from build123d import *

# Parameters (mm, degrees)
SZKIC1_W                       = 40
SZKIC1_H                       = 14
SZKIC1_R                       = 2
DODANIE_WYCI_GNI_CIE1_DEPTH    = 10.77
SZKIC2_W                       = 56
SZKIC2_H                       = 14
DODANIE_WYCI_GNI_CIE2_DEPTH    = 20.3
SZKIC5_R                       = 2.25
WYTNIJ_WYCI_GNI_CIE2_DEPTH     = 14
SZKIC8_W                       = 56
SZKIC8_H                       = 10.77
DODANIE_WYCI_GNI_CIE3_DEPTH    = 14
WYTNIJ_WYCI_GNI_CIE3_START     = -14
WYTNIJ_WYCI_GNI_CIE3_OUTLINE_W = 42
WYTNIJ_WYCI_GNI_CIE3_OUTLINE_H = 21
WYTNIJ_WYCI_GNI_CIE3_DEPTH     = 14
SZKIC12_R                      = 2.25
DODANIE_WYCI_GNI_CIE4_DEPTH    = 18
WYTNIJ_WYCI_GNI_CIE1_DEPTH     = 5
SZKIC9_R                       = 2.2
WYTNIJ_WYCI_GNI_CIE4_DEPTH     = 21
SZKIC10_W                      = 56
SZKIC10_H                      = 21
WYTNIJ_WYCI_GNI_CIE5_DEPTH     = 17
SZKIC13_W                      = 21
SZKIC13_H                      = 15
DODANIE_WYCI_GNI_CIE5_DEPTH    = 0.7
SZKIC16_W                      = 21
SZKIC16_H                      = 15
DODANIE_WYCI_GNI_CIE7_DEPTH    = 0.7


# Read off the part's stored shape, not the designer's step: Wytnij-wyciągnięcie3
with BuildPart() as part:
    # Szkic1 → Dodanie-wyciągnięcie1 (new body)
    with BuildSketch(Plane.XY):
        Rectangle(SZKIC1_W, SZKIC1_H)
        with Locations((-14, 0)):
            Circle(SZKIC1_R, mode=Mode.SUBTRACT)
        with Locations((14, 0)):
            Circle(SZKIC1_R, mode=Mode.SUBTRACT)
    extrude(amount=DODANIE_WYCI_GNI_CIE1_DEPTH)

    # Szkic2 → Dodanie-wyciągnięcie2 (add)
    with BuildSketch(Plane.XY.offset(10.77)):
        Rectangle(SZKIC2_W, SZKIC2_H)
    extrude(amount=DODANIE_WYCI_GNI_CIE2_DEPTH)

    # Szkic5 → Wytnij-wyciągnięcie2 (cut)
    with BuildSketch(Plane(origin=(0, 7, 0), x_dir=(1, 0, 0), z_dir=(0, 1, 0))):
        with Locations(Location((-24, -15.92, 0), (0, 0, 180))):
            Circle(SZKIC5_R)
        with Locations(Location((24, -15.92, 0), (0, 0, 180))):
            Circle(SZKIC5_R)
        with Locations(Location((24, -25.92, 0), (0, 0, 180))):
            Circle(SZKIC5_R)
        with Locations(Location((-24, -25.92, 0), (0, 0, 180))):
            Circle(SZKIC5_R)
    extrude(amount=-WYTNIJ_WYCI_GNI_CIE2_DEPTH, mode=Mode.SUBTRACT)

    # Szkic8 → Dodanie-wyciągnięcie3 (add)
    with BuildSketch(Plane(origin=(0, 7, 0), x_dir=(1, 0, 0), z_dir=(0, 1, 0))):
        with Locations((0, -5.385)):
            Rectangle(SZKIC8_W, SZKIC8_H)
    extrude(amount=-DODANIE_WYCI_GNI_CIE3_DEPTH)

    # Wytnij-wyciągnięcie3 outline → Wytnij-wyciągnięcie3 (cut)
    with BuildSketch(Plane(origin=(0, 7, 0), x_dir=(1, 0, 0), z_dir=(0, 1, 0)).offset(WYTNIJ_WYCI_GNI_CIE3_START)):
        with Locations((-0.124911353, -20.57)):
            Rectangle(WYTNIJ_WYCI_GNI_CIE3_OUTLINE_W, WYTNIJ_WYCI_GNI_CIE3_OUTLINE_H)
    extrude(amount=WYTNIJ_WYCI_GNI_CIE3_DEPTH, mode=Mode.SUBTRACT)

    # Szkic12 → Dodanie-wyciągnięcie4 (add)
    with BuildSketch(Plane.XZ.offset(7)):
        Polygon((20.875088647, 31.07), (20.875088647, 10.07), (-21.124911353, 10.07), (-21.124911353, 31.07), (-28, 31.07), (-28, 0), (28, 0), (28, 31.07), align=None)
        with Locations(Location((-24, 25.92, 0), (0, 0, 180))):
            Circle(SZKIC12_R, mode=Mode.SUBTRACT)
        with Locations(Location((24, 25.92, 0), (0, 0, 180))):
            Circle(SZKIC12_R, mode=Mode.SUBTRACT)
        with Locations(Location((-24, 15.92, 0), (0, 0, 180))):
            Circle(SZKIC12_R, mode=Mode.SUBTRACT)
        with Locations(Location((24, 15.92, 0), (0, 0, 180))):
            Circle(SZKIC12_R, mode=Mode.SUBTRACT)
    extrude(amount=DODANIE_WYCI_GNI_CIE4_DEPTH)

    # Szkic4 → Wytnij-wyciągnięcie1 (cut)
    with BuildSketch(Plane.XY.offset(10.77)):
        Polygon((-16.078460969, 3.6), (-18.156921938, 0), (-16.078460969, -3.6), (-11.921539031, -3.6), (-9.843078062, 0), (-11.921539031, 3.6), align=None)
        Polygon((11.921539031, 3.6), (9.843078062, 0), (11.921539031, -3.6), (16.078460969, -3.6), (18.156921938, 0), (16.078460969, 3.6), align=None)
    extrude(amount=-WYTNIJ_WYCI_GNI_CIE1_DEPTH, mode=Mode.SUBTRACT)

    # Szkic9 → Wytnij-wyciągnięcie4 (cut)
    with BuildSketch(Plane.XY.offset(10.07)):
        with Locations((-14, 0)):
            Circle(SZKIC9_R)
        with Locations((14, 0)):
            Circle(SZKIC9_R)
    extrude(amount=-WYTNIJ_WYCI_GNI_CIE4_DEPTH, mode=Mode.SUBTRACT)

    # Szkic10 → Wytnij-wyciągnięcie5 (cut)
    with BuildSketch(Plane(origin=(0, 7, 0), x_dir=(1, 0, 0), z_dir=(0, 1, 0))):
        with Locations((0, -20.57)):
            Rectangle(SZKIC10_W, SZKIC10_H)
    extrude(amount=-WYTNIJ_WYCI_GNI_CIE5_DEPTH, mode=Mode.SUBTRACT)

    # Szkic13 → Dodanie-wyciągnięcie5 (add)
    with BuildSketch(Plane(origin=(-21.124911353, 0, 0), x_dir=(0, 0, -1), z_dir=(1, 0, 0))):
        with Locations((-20.57, -17.5)):
            Rectangle(SZKIC13_W, SZKIC13_H)
    extrude(amount=DODANIE_WYCI_GNI_CIE5_DEPTH)

    # Szkic16 → Dodanie-wyciągnięcie7 (add)
    with BuildSketch(Plane.ZY.offset(-20.875088647)):
        with Locations((20.57, -17.5)):
            Rectangle(SZKIC16_W, SZKIC16_H)
    extrude(amount=DODANIE_WYCI_GNI_CIE7_DEPTH)


solid = part.part
CAD build for the part. Positions are in the model's coordinates, mm. A direction names the side the tool comes from. Coordinates: 2 decimals unless noted, no trailing zeros. Order: outer loops, then holes, each group sorted by start corner. A loop starts at its lowest first (then second) coordinate and runs counter-clockwise, first axis right, second up.
Item 1: 3-axis set-ups, long thin cutter, end or side, ignore diameter. For faces 5 (the face through (-28, -12, 12)), 6 (the face through (-14, -3.6, 8)), 7 (the face through (-24, -10, 21)): which of +Z, -Z, +X, -X, +Y, -Y reach the whole face in a straight line?
Check sheet entries:
face 5: +Z, -Z, -X, +Y, -Y
face 6: +Z
face 7: +Z, +X, -X, +Y
Item 2: Drill centre lines: L1, parallel to Z at x = -24, y = -21.25; L2, parallel to X at y = -21.5, z = 25.92; L3, parallel to Z at x = -24.5, y = -14. Where is each one in solid material? Low to high.
Check sheet entries:
L1: z = 0 to 13.67, 18.17 to 23.67, 28.17 to 31.07
L2: x = -28 to -26.25, -21.75 to -20.42, 20.18 to 21.75, 26.25 to 28
L3: z = 0 to 13.73, 18.11 to 23.73, 28.11 to 31.07
Item 3: Band-saw the part on D-D on y = -17. List the corners of the cut face in (x, z).
Check sheet entries:
outline: (-28, 0) - (28, 0) - (28, 31.07) - (20.18, 31.07) - (20.18, 10.07) - (-20.42, 10.07) - (-20.42, 31.07) - (-28, 31.07) - close; hole circle Ø4.5 at (-24, 15.92); hole circle Ø4.5 at (-24, 25.92); hole circle Ø4.5 at (24, 15.92); hole circle Ø4.5 at (24, 25.92)
Item 4: Band-saw the part on C-C on x = 14. List the corners of the cut face in (y, z), plus the area to 3 significant figures.
Check sheet entries:
outline: (-25, 0) - (-2.2, 0) - (-2.2, 5.77) - (-3.6, 5.77) - (-3.6, 10.07) - (-25, 10.07) - close; (2.2, 0) - (7, 0) - (7, 10.07) - (3.6, 10.07) - (3.6, 5.77) - (2.2, 5.77) - close
area: 266 mm2
Item 5: Band-saw the part on B-B on z = 25.92. List the corners of the cut face in (x, y), plus the area to 3 significant figures.
Check sheet entries:
outline: (-28, -25) - (-26.25, -25) - (-26.25, -10) - (-28, -10) - close; (-21.75, -25) - (-20.42, -25) - (-20.42, -10) - (-21.75, -10) - close; (20.18, -25) - (21.75, -25) - (21.75, -10) - (20.18, -10) - close; (26.25, -25) - (28, -25) - (28, -10) - (26.25, -10) - close
area: 96.0 mm2
Item 6: Pin check, flat tips, straight feed: pin 1 Ø2 at (x, z) = (22, 17) entering from +Y; pin 2 Ø5 at (x, y) = (-15.5, -8.5) entering from +Z. Stop position of each tip, or through.
Check sheet entries:
pin 1: stops at y = -10
pin 2: stops at z = 10.07
Item 7: Band-saw the part on A-A on x = -24. List the corners of the cut face in (y, z).
Check sheet entries:
outline: (-25, 0) - (7, 0) - (7, 10.07) - (-10, 10.07) - (-10, 13.67) - (-25, 13.67) - close; (-25, 18.17) - (-10, 18.17) - (-10, 23.67) - (-25, 23.67) - close; (-25, 28.17) - (-10, 28.17) - (-10, 31.07) - (-25, 31.07) - close
Item 8: Two-plate mould, pull along Z, no slides. Class faces 1 (the face through (22.79, -17.395, 24.023)), 2 (the face through (24, -18, 31.07)), 3 (the face through (-26.146, -17.395, 15.244)), 4 (the face through (24, -10, 20)): +Z half, -Z half, draft (parallel to the pull), parting line (faces both ways), or undercut.
Check sheet entries:
face 1: undercut
face 2: +Z half
face 3: undercut
face 4: draft
